Geometry check sheet. Reference: the model listing, model coordinates, mm. A direction names the side the tool comes from. Coordinates: 2 decimals unless noted, no trailing zeros. Loops run counter-clockwise (first coordinate to the right, second up) from the corner with the lowest first, then second, coordinate; pieces in that order, holes last. Notation, with made-up numbers: M 35.5,74 L 78.5,74 A13 cw 78.5,79 Z; hole C 28,-31.5 d6. An arc over 180 degrees is marked long. Use CSV: the item, a comma, the result in double quotes.
```python
from build123d import *

# Parameters (mm, degrees)
SKETCH_1_W           = 590
SKETCH_1_H           = 11.5
EXTRUDE_1_DEPTH      = 5
SKETCH_2_W           = 590
SKETCH_2_H           = 8.5
CUT_EXTRUDE_1_DEPTH  = 3.5
SKETCH_3_W           = 390
SKETCH_3_H           = 11.5
EXTRUDE_2_DEPTH      = 10
CHAMFER_1_SIZE       = 10
CUT_EXTRUDE_2_DEPTH  = 296.604888322
SKETCH_5_W           = 377.928932188
SKETCH_5_H           = 8.5
CUT_EXTRUDE_3_DEPTH  = 3.5
SKETCH_7_W           = 9.262731361
SKETCH_7_H           = 8.5
CUT_EXTRUDE_5_DEPTH  = 2.5
SKETCH_8_W           = 5
SKETCH_8_H           = 200
EXTRUDE_3_DEPTH      = 20
CUT_EXTRUDE_6_DEPTH  = 297.29050356
CUT_EXTRUDE_7_DEPTH  = 297.29050356
CUT_EXTRUDE_8_DEPTH  = 3.5
SKETCH_12_W          = 5
SKETCH_12_H          = 300
EXTRUDE_4_DEPTH      = 30
CUT_EXTRUDE_9_DEPTH  = 298.536657405
CUT_EXTRUDE_10_DEPTH = 3.5
SKETCH_16_R          = 1.5
CUT_EXTRUDE_11_DEPTH = 298.536657405


with BuildPart() as part:
    # 草图1 → 凸台-拉伸1 (new body)
    with BuildSketch(Plane(origin=(0, 0, 0), x_dir=(0, 0, -1), z_dir=(1, 0, 0))):
        Rectangle(SKETCH_1_W, SKETCH_1_H)
    extrude(amount=EXTRUDE_1_DEPTH)

    # 草图2 → 切除-拉伸1 (cut)
    with BuildSketch(Plane.ZY):
        with Locations((0, -0.131137871)):
            Rectangle(SKETCH_2_W, SKETCH_2_H)
    extrude(amount=-CUT_EXTRUDE_1_DEPTH, mode=Mode.SUBTRACT)

    # 草图3 → 凸台-拉伸2 (add)
    with BuildSketch(Plane(origin=(5, 0, 0), x_dir=(0, 0, -1), z_dir=(1, 0, 0))):
        with Locations((100, 0)):
            Rectangle(SKETCH_3_W, SKETCH_3_H)
    extrude(amount=EXTRUDE_2_DEPTH)

    # 倒角1
    chamfer_1_edges = [part.edges().sort_by_distance(p)[0] for p in [
        (15, 0, 95),
    ]]
    chamfer(chamfer_1_edges, length=CHAMFER_1_SIZE - 0.0001)  # a hair under: the kernel refuses the full size

    # 草图4 → 切除-拉伸2 (cut, through all)
    with BuildSketch(Plane(origin=(0, 5.75, 0), x_dir=(1, 0, 0), z_dir=(0, 1, 0))):
        Polygon((0, -92.928932188), (0, 295), (10, 295), (10, -82.928932188), align=None)
    extrude(amount=-CUT_EXTRUDE_2_DEPTH, mode=Mode.SUBTRACT)

    # 草图5 → 切除-拉伸3 (cut)
    with BuildSketch(Plane.ZY.offset(-10)):
        with Locations((-106.035533906, 0)):
            Rectangle(SKETCH_5_W, SKETCH_5_H)
    extrude(amount=-CUT_EXTRUDE_3_DEPTH, mode=Mode.SUBTRACT)

    # 草图7 → 切除-拉伸5 (cut)
    with BuildSketch(Plane(origin=(46.464466094, 0, 46.464466094), x_dir=(-0.7071067811865471, 0, 0.7071067811865479), z_dir=(-0.7071067811865479, 0, -0.7071067811865471))):
        with Locations((61.079312439, -0.131137871)):
            Rectangle(SKETCH_7_W, SKETCH_7_H)
    extrude(amount=-CUT_EXTRUDE_5_DEPTH, mode=Mode.SUBTRACT)

    # 草图8 → 凸台-拉伸3 (add)
    with BuildSketch(Plane(origin=(0, 5.75, 0), x_dir=(1, 0, 0), z_dir=(0, 1, 0))):
        with Locations((2.5, -195)):
            Rectangle(SKETCH_8_W, SKETCH_8_H)
    extrude(amount=EXTRUDE_3_DEPTH)

    # 草图9 → 切除-拉伸6 (cut, through all)
    with BuildSketch(Plane(origin=(5, 0, 0), x_dir=(0, 0, -1), z_dir=(1, 0, 0))):
        Polygon((-295, 14.25), (-131.790247395, 14.25), (-95, -5.75), (-295, -5.75), align=None)
    extrude(amount=-CUT_EXTRUDE_6_DEPTH, mode=Mode.SUBTRACT)

    # 草图10 → 切除-拉伸7 (cut, through all)
    with BuildSketch(Plane(origin=(5, 0, 0), x_dir=(0, 0, -1), z_dir=(1, 0, 0))):
        Polygon((-95, 5.75), (-131.790247395, 25.75), (-95, 25.75), align=None)
    extrude(amount=-CUT_EXTRUDE_7_DEPTH, mode=Mode.SUBTRACT)

    # 草图11 → 切除-拉伸8 (cut)
    with BuildSketch(Plane.ZY):
        Polygon((132.171609821, 24.25), (95.140132691, 4.118862129), (110.013262981, 4.118862129), (131.408884969, 15.75), (295, 15.75), (295, 24.25), align=None)
    extrude(amount=-CUT_EXTRUDE_8_DEPTH, mode=Mode.SUBTRACT)

    # 草图12 → 凸台-拉伸4 (add)
    with BuildSketch(Plane(origin=(0, 5.75, 0), x_dir=(1, 0, 0), z_dir=(0, 1, 0))):
        with Locations((12.5, 145)):
            Rectangle(SKETCH_12_W, SKETCH_12_H)
    extrude(amount=EXTRUDE_4_DEPTH)

    # 草图13 → 切除-拉伸9 (cut, through all)
    with BuildSketch(Plane(origin=(15, 0, 0), x_dir=(0, 0, -1), z_dir=(1, 0, 0))):
        Polygon((-1.619558014, -5.75), (45, 24.25), (295, 24.25), (295, -5.75), align=None)
        Polygon((-5, 5.75), (41.619558014, 35.75), (-5, 35.75), align=None)
    extrude(amount=-CUT_EXTRUDE_9_DEPTH, mode=Mode.SUBTRACT)

    # 草图15 → 切除-拉伸10 (cut)
    with BuildSketch(Plane.ZY.offset(-10)):
        Polygon((-44.559072784, 25.75), (-295, 25.75), (-295, 34.25), (-42.06048523, 34.25), (4.559072784, 4.25), (-11.148389541, 4.25), align=None)
    extrude(amount=-CUT_EXTRUDE_10_DEPTH, mode=Mode.SUBTRACT)

    # 草图16 → 切除-拉伸11 (cut, through all)
    with BuildSketch(Plane(origin=(15, 0, 0), x_dir=(0, 0, -1), z_dir=(1, 0, 0))):
        with Locations((160, 30)):
            Circle(SKETCH_16_R)
        with Locations((265, 30)):
            Circle(SKETCH_16_R)
    extrude(amount=-CUT_EXTRUDE_11_DEPTH, mode=Mode.SUBTRACT)


solid = part.part
```
1. Release check for a two-part mould opening along Y. For faces 1 (the flat face through (2.54, 15.61, 113.14)), 2 (the flat face through (3.5, 17, 194)), 3 (the flat face through (10, 0, 90)), 4 (the flat face through (13.5, 28, -107)) record: +Y half, -Y half, draft (parallel to the pull), parting line (faces both ways), or undercut.
The answers:
face 1,"+Y half"
face 2,"undercut"
face 3,"draft"
face 4,"undercut"
2. Section check A-A, the plane z = 49.5. Record the cut outline in (x, y).
The answers:
outline,"M 10,-5.75 L 15,-5.75 L 15,5.75 L 10,5.75 L 10,4.25 L 13.5,4.25 L 13.5,-4.25 L 10,-4.25 Z"
3. Thickness scan on line 1 (Y direction, x = 13.9, z = -265); line 2 (Y direction, x = 2.5, z = 257.5); line 3 (X direction, y = 24.5, z = 137). Record the ranges inside material, lowest first. Write a range as [from, to].
The answers:
line 1,"[24.25, 28.5], [31.5, 35.75]"
line 2,"[14.25, 15.75], [24.25, 25.75]"
line 3,"[0, 5]"
4. Set-up check for faces 5 (the flat face through (10, 35, -105)), 6 (the flat face through (0, 15, 203)), 7 (the flat face through (1.726, 9.853, 120.561)): record each of +Z, -Z, +X, -X, +Y, -Y from which the full face is reachable in a straight line by a thin tool's end or side.
The answers:
face 5,"-Z, -X, +Y, -Y"
face 6,"+Z, -Z, -X, +Y, -Y"
face 7,"-X"
5. Gauge pin test, flat ends, axial feed: P1, Ø1.6, axis at x = 1.5, z = 112, coming from the -Y side; P2, Ø4, axis at x = 12, z = 36, coming from the +Y side; P3, Ø4, axis at x = 13.5, z = -197, coming from the -Y side. Record the tip position at first contact, or that the pin passes through.
The answers:
P1,"y = 4.12"
P2,"y = 5.75"
P3,"y = 24.25"
